Check sheet for the modelled part. Datum: model origin and axes. Units: mm. Give positions to 0.01 mm unless a question says otherwise; leave off trailing zeros. Write each loop counter-clockwise with the first axis right and the second up, starting at its lowest first coordinate (ties: lowest second). Pieces come first, ordered by that corner, then holes. Notation, with made-up numbers: M -34,-6.5 L 17,-6.5 A29 ccw 17,27.5 Z; hole C 85.25,75 d9. An arc over 180 degrees is marked long. Write item = value, one per line. Start each with the question number.
1) Cross-section at C-C, the plane z = 1.3. Record the cut outline in (x, y).
2) Go/stop test with flat-tipped pins: pin 1 (2.5 mm diameter, centred on x = -7.5, y = -19, fed in from -Z); pin 2 (1.5 mm diameter, centred on x = -2.5, z = 0.5, fed in from -Y). Record where each tip stops, or that it passes through.
3) Cross-section at A-A, the plane y = -19. Record the cut outline in (x, z), plus the area to 3 significant figures.
4) Cross-section at B-B, the plane x = 0. Record the cut outline in (y, z).
5) Scan lines: line 1 along X through (y, z) = (-33.5, 0.55); line 2 along Y through (x, z) = (7.75, 1.9); line 3 along Y through (x, z) = (6.75, 0.7). Record each from-to range of solid material in increasing order. Write a range as [from, to].
```python
from build123d import *

# Parameters (mm, degrees)
SKETCH_1_R          = 9.5
EXTRUDE_1_DEPTH     = 3
FILLET_START        = -1
FILLET_2_DEPTH      = 5
SKETCH_2_R          = 2
CUT_EXTRUDE_1_DEPTH = 10


with BuildPart() as part:
    # 草图1 → 凸台-拉伸1 (new body)
    with BuildSketch(Plane.XY):
        with BuildLine():
            Line((-15, 0), (-15, -120))
            ThreePointArc((-15, -120), (0, -135), (15, -120))
            Line((15, -120), (15, 0))
            ThreePointArc((15, 0), (0, -15), (-15, 0))
        make_face()
        with Locations((0, -120)):
            Circle(SKETCH_1_R, mode=Mode.SUBTRACT)
    extrude(amount=EXTRUDE_1_DEPTH)

    # 圆角2: read off the stored shape, not the designer's step
    # 圆角2 outline → 圆角2 (cut)
    with BuildSketch(Plane.XY.offset(FILLET_START)):
        with BuildLine():
            Line((-15, 0), (-15, -17.320508076))
            ThreePointArc((-15, -17.320508076), (-12.5, -12.990381057), (-7.5, -12.990381057))
            ThreePointArc((-7.5, -12.990381057), (-12.990381057, -7.5), (-15, 0))
        make_face()
        with BuildLine():
            ThreePointArc((15, 0), (12.990381057, -7.5), (7.5, -12.990381057))
            ThreePointArc((7.5, -12.990381057), (12.5, -12.990381057), (15, -17.320508076))
            Line((15, -17.320508076), (15, 0))
        make_face()
    extrude(amount=FILLET_2_DEPTH, mode=Mode.SUBTRACT)

    # 草图2 → 切除-拉伸1 (cut)
    with BuildSketch(Plane.XY.offset(3)):
        with Locations((-7.5, -19)):
            Circle(SKETCH_2_R)
        with Locations((-7.5, -33)):
            Circle(SKETCH_2_R)
        with Locations((7.5, -33)):
            Circle(SKETCH_2_R)
        with Locations((7.5, -19)):
            Circle(SKETCH_2_R)
    extrude(amount=-CUT_EXTRUDE_1_DEPTH, mode=Mode.SUBTRACT)


solid = part.part
```
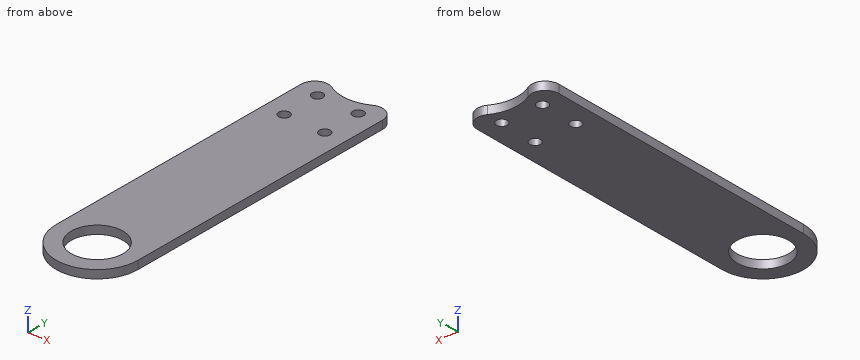
Reply:
q1.outline = M -15,-120 A15 ccw 15,-120 L 15,-17.32 A5 ccw 7.5,-12.99 A15 cw -7.5,-12.99 A5 ccw -15,-17.32 Z; hole C 0,-120 d19; hole C -7.5,-33 d4; hole C -7.5,-19 d4; hole C 7.5,-33 d4; hole C 7.5,-19 d4
q2.pin_1 = through
q2.pin_2 = -134.9
q3.outline = M -15,0 L -9.5,0 L -9.5,3 L -15,3 Z; M -5.5,0 L 5.5,0 L 5.5,3 L -5.5,3 Z; M 9.5,0 L 15,0 L 15,3 L 9.5,3 Z
q3.area = 66.0 mm2
q4.outline = M -135,0 L -129.5,0 L -129.5,3 L -135,3 Z; M -110.5,0 L -15,0 L -15,3 L -110.5,3 Z
q5.line_1 = [-15, -9.44], [-5.56, 5.56], [9.44, 15]
q5.line_2 = [-132.84, -125.49], [-114.51, -34.98], [-31.02, -20.98], [-17.02, -12.86]
q5.line_3 = [-133.4, -126.68], [-113.32, -34.85], [-31.15, -20.85], [-17.15, -13.4]
